```python
from build123d import *

# Parameters (mm, degrees)
SKETCH_1_W          = 60
SKETCH_1_H          = 30
SKETCH_1_R          = 4
EXTRUDE_1_DEPTH     = 4
SKETCH_2_W          = 7
SKETCH_2_H          = 30
EXTRUDE_2_DEPTH     = 30
SKETCH_4_W          = 7
SKETCH_4_H          = 78.572897546
EXTRUDE_3_DEPTH     = 27.51
FILLET_1_R          = 16
CUT_EXTRUDE_2_DEPTH = 89.228478483
FILLET_2_R          = 15


with BuildPart() as part:
    # 草圖1 → 填料-伸長1 (new body)
    with BuildSketch(Plane(origin=(0, 0, 0), x_dir=(1, 0, 0), z_dir=(0, 1, 0))):
        Rectangle(SKETCH_1_W, SKETCH_1_H)
        with Locations(Location((15, 0, 0), (0, 0, 270))):
            Circle(SKETCH_1_R, mode=Mode.SUBTRACT)
    extrude(amount=EXTRUDE_1_DEPTH)

    # 草圖2 → 填料-伸長2 (add)
    with BuildSketch(Plane(origin=(0, 4, 0), x_dir=(1, 0, 0), z_dir=(0, 1, 0))):
        with Locations((-26.5, 0)):
            Rectangle(SKETCH_2_W, SKETCH_2_H)
    extrude(amount=EXTRUDE_2_DEPTH)

    # 草圖4 → 填料-伸長3 (add)
    with BuildSketch(Plane(origin=(0, 0, -15), x_dir=(-1, 0, 0), z_dir=(0, 0, -1))):
        with Locations((26.5, 17)):
            Rectangle(SKETCH_4_W, SKETCH_4_H)
    extrude_3 = extrude(amount=EXTRUDE_3_DEPTH)

    # 鏡射1: 填料-伸長3 across plane
    add(extrude_3.mirror(Plane.XY))

    # 圓角1
    fillet_1_edges = [part.edges().sort_by_distance(p)[0] for p in [
        (-23, 4, 0),
    ]]
    fillet(fillet_1_edges, radius=FILLET_1_R)

    # 草圖5 → 除料-伸長2 (cut, through all)
    with BuildSketch(Plane(origin=(-23, 0, 0), x_dir=(0, 0, -1), z_dir=(1, 0, 0))):
        with BuildLine():
            Line((21.01, 19.5), (34.01, 19.5))
            ThreePointArc((34.01, 19.5), (36.51, 17), (34.01, 14.5))
            Line((34.01, 14.5), (21.01, 14.5))
            ThreePointArc((21.01, 14.5), (18.51, 17), (21.01, 19.5))
        make_face()
    extrude(amount=-CUT_EXTRUDE_2_DEPTH, mode=Mode.SUBTRACT)

    # 圓角2
    fillet_2_edges = [part.edges().sort_by_distance(p)[0] for p in [
        (30, 2, 15),
        (30, 2, -15),
    ]]
    fillet(fillet_2_edges, radius=FILLET_2_R - 0.0001)  # a hair under: the kernel refuses the full size


solid = part.part
```
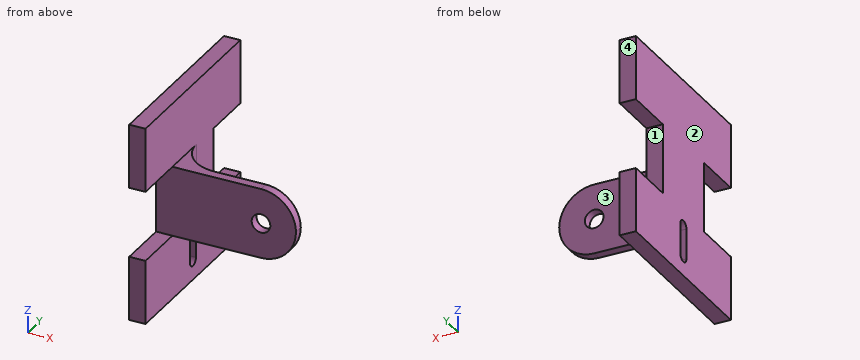
Could you check a few things on this model? Use its own coordinates, in mm. Face numbers are marked on the shaded views. A direction names the side the tool comes from. Round coordinates to 2 decimals unless told otherwise and drop trailing zeros. Loops run counter-clockwise (first coordinate to the right, second up) from the corner with the lowest first, then second, coordinate; pieces in that order, holes last. Notation, with made-up numbers: (-39, 83.5) - (-28, 83.5) arc R23 ccw to (-28, 97.5) - close; hole circle Ø4 at (25, -37). An arc over 180 degrees is marked (long way). Use CSV: the item, a comma, the result in double quotes.
Item 1: If we section it at D-D on z = 7: List the corners of the cut face in (x, y) for me.
Here are the results:
outline,"(-30, 0) - (28.27, 0) - (28.27, 4) - (-7, 4) arc R16 cw to (-23, 20) - (-23, 34) - (-30, 34) - close"
Item 2: If we section it at B-B on y = 44: List the corners of the cut face in (x, z) for me.
Here are the results:
outline,"(-30, -42.51) - (-23, -42.51) - (-23, -15) - (-30, -15) - close; (-30, 15) - (-23, 15) - (-23, 42.51) - (-30, 42.51) - close"
Item 3: If we mould it in two halves opening along Z, with no side actions, what happens to the marked faces 1 and 2? For each: pulls with the +Z half, pulls with the -Z half, needs draft (parallel to the pull), parting line crosses it, or undercut.
Here are the results:
face 1,"undercut"
face 2,"needs draft"
Item 4: If we section it at A-A on x = -26: List the corners of the cut face in (y, z) for me.
Here are the results:
outline,"(-22.29, -42.51) - (56.29, -42.51) - (56.29, -15) - (34, -15) - (34, 15) - (56.29, 15) - (56.29, 42.51) - (-22.29, 42.51) - (-22.29, 15) - (0, 15) - (0, -15) - (-22.29, -15) - close; hole (14.5, -34.01) arc R2.5 ccw to (19.5, -34.01) - (19.5, -21.01) arc R2.5 ccw to (14.5, -21.01) - close"
Item 5: I need wall thicknesses on L1, parallel to Y at x = -27.5, z = -26.5; L2, parallel to Z at x = -27, y = 38; L3, parallel to X at y = 2, z = 0. Which ranges of each line are inside material? Lowest first, please. Write a range as [from, to].
Here are the results:
L1,"y = [-22.29, 14.5], [19.5, 56.29]"
L2,"z = [-42.51, -15], [15, 42.51]"
L3,"x = [-30, 11], [19, 30]"
Item 6: For the marked faces 3 and 4, which set-ups out of +Z, -Z, +X, -X, +Y, -Y let a thin tool reach every point of the face, with its end or its side?
Here are the results:
face 3,"+Z, -Z, +X, +Y"
face 4,"+Z, -Z, +X, -X, +Y"
Item 7: If we section it at C-C on y = 10: List the corners of the cut face in (x, z) for me, then the cut area to 3 significant figures.
Here are the results:
outline,"(-30, -42.51) - (-23, -42.51) - (-23, -15) - (-19.49, -15) - (-19.49, 15) - (-23, 15) - (-23, 42.51) - (-30, 42.51) - close"
area,"700 mm²"
Item 8: Will these pins go through, and if not, where does the flat tip stop? pin 1 (22 mm diameter, centred on x = -3, y = 8, fed in from -Z); pin 2 (12 mm diameter, centred on x = 23, z = 12.5, fed in from +Y); pin 3 (2 mm diameter, centred on x = -10.5, y = 0, fed in from +Z).
Here are the results:
pin 1,"stops at z = -15"
pin 2,"stops at y = 4"
pin 3,"stops at z = 15"
